Build history of the part. All positions in model axes, mm. Coordinates: 2 decimals unless noted, no trailing zeros. Order: outer loops, then holes, each group sorted by start corner. A loop starts at its lowest first (then second) coordinate and runs counter-clockwise, first axis right, second up. Notation, with made-up numbers: (23.25, -26.75) -> (40.25, -26.75) arc R26 ccw to (40.25, -9.75) -> close; hole circle Ø7 at (41.5, -0.75). An arc over 180 degrees is marked (long way). Write each question's results on one line, items separated by ' | '.
from build123d import *

# Parameters (mm, degrees)
SKETCH1_R           = 9.9
BOSS_EXTRUDE1_DEPTH = 75
CHAMFER1_SIZE       = 1
CHAMFER2_SIZE       = 1


with BuildPart() as part:
    # Sketch1 → Boss-Extrude1 (new body)
    with BuildSketch(Plane.XY):
        Circle(SKETCH1_R)
    extrude(amount=BOSS_EXTRUDE1_DEPTH)

    # Chamfer1
    chamfer1_edges = [part.edges().sort_by_distance(p)[0] for p in [
        (-9.9, 0, 0),
    ]]
    chamfer(chamfer1_edges, length=CHAMFER1_SIZE)

    # Chamfer2
    chamfer2_edges = [part.edges().sort_by_distance(p)[0] for p in [
        (-9.9, 0, 75),
    ]]
    chamfer(chamfer2_edges, length=CHAMFER2_SIZE)


solid = part.part
Item 1: Drill centre lines: line 1 (X direction, y = -0.5, z = 31); line 2 (Z direction, x = -8.5, y = 2.75); line 3 (X direction, y = 1.25, z = 13.5). Where is each one in solid material? Low to high. Write a range as from..to.
Answer:
line 1: x = -9.89..9.89 | line 2: z = 0.03..74.97 | line 3: x = -9.82..9.82
Item 2: Slice it at A-A, the plane z = 51. List the corners of the cut face in (x, y).
Answer:
outline: circle Ø19.8 at (0, 0)
Item 3: Pin check, flat tips, straight feed: pin 1 (10 mm diameter, centred on y = -1.5, z = 63, fed in from +X); pin 2 (5 mm diameter, centred on y = -7.5, z = 32, fed in from -X); pin 3 (2 mm diameter, centred on x = 5.5, z = 50, fed in from +Y); pin 4 (3 mm diameter, centred on x = 4.5, z = 38, fed in from -Y). Stop position of each tip, or through.
Answer:
pin 1: stops at x = 9.9 | pin 2: stops at x = -8.54 | pin 3: stops at y = 8.82 | pin 4: stops at y = -9.43
